CAD build for the part. Positions are in the model's coordinates, mm. A direction names the side the tool comes from. Round coordinates to 2 decimals unless told otherwise and drop trailing zeros. Write each loop counter-clockwise with the first axis right and the second up, starting at its lowest first coordinate (ties: lowest second). Pieces come first, ordered by that corner, then holes. Notation, with made-up numbers: (54.25, 57) - (62.25, 57) arc R30 ccw to (62.25, 94) - close; hole circle Ø5 at (-35, -18.5). An arc over 180 degrees is marked (long way). Answer in a Markdown table with one row per item.
```python
from build123d import *

# Parameters (mm, degrees)
F0_W     = 6.35
F0_H     = 38.1
F1_DEPTH = 25.4
F3_DEPTH = 12.5


with BuildPart() as f1:
    # F0 (on Top) → F1 (new body)
    with BuildSketch(Plane.XY):
        with Locations((-3.175, 0)):
            Rectangle(F0_W, F0_H)
    extrude(amount=F1_DEPTH)

    # F2 (on face) → F3 (join)
    with BuildSketch(Plane(origin=(-6.35, 0, 0), x_dir=(0, -1, 0), z_dir=(-1, 0, 0))):
        with BuildLine():
            Line((-19.05, 25.4), (-19.05, 19.05))
            ThreePointArc((-19.05, 19.05), (0, 0), (19.05, 19.05))
            Line((19.05, 19.05), (19.05, 25.4))
            Line((19.05, 25.4), (14, 25.4))
            Line((14, 25.4), (14, 19.05))
            ThreePointArc((14, 19.05), (0, 5.05), (-14, 19.05))
            Line((-14, 19.05), (-14, 25.4))
            Line((-14, 25.4), (-19.05, 25.4))
        make_face()
    extrude(amount=F3_DEPTH)


solid = f1.part
```
Q1. Saw through at C-C on z = 9.5. List the corners of the cut face in (x, y), then the cut area to 3 significant figures.
Computed:
| item | result |
|---|---|
| outline | (-18.85, -16.48) - (-6.35, -16.48) - (-6.35, -19.05) - (0, -19.05) - (0, 19.05) - (-6.35, 19.05) - (-6.35, 16.48) - (-18.85, 16.48) - (-18.85, 10.24) - (-6.35, 10.24) - (-6.35, -10.24) - (-18.85, -10.24) - close |
| area | 398 mm2 |
Q2. 3-axis set-ups, long thin cutter, end or side, ignore diameter. For faces 1 (the flat face through (-6.35, 14, 4)), 2 (the flat face through (-6.35, -15, 5)), 3 (the cylindrical face through (-13, 0, 0)), 4 (the cylindrical face through (-12.512, -0.308, 5.053)): which of +Z, -Z, +X, -X, +Y, -Y reach the whole face in a straight line?
Computed:
| item | result |
|---|---|
| face 1 | -Z, -X, +Y |
| face 2 | -Z, -X, -Y |
| face 3 | -Z, -X |
| face 4 | +Z, -X |
Q3. Saw through at D-D on z = 17.5. List the corners of the cut face in (x, y).
Computed:
| item | result |
|---|---|
| outline | (-18.85, -18.99) - (-6.35, -18.99) - (-6.35, -19.05) - (0, -19.05) - (0, 19.05) - (-6.35, 19.05) - (-6.35, 18.99) - (-18.85, 18.99) - (-18.85, 13.91) - (-6.35, 13.91) - (-6.35, -13.91) - (-18.85, -13.91) - close |
Q4. Saw through at B-B on x = -7.75. List the corners of the cut face in (y, z).
Computed:
| item | result |
|---|---|
| outline | (-19.05, 19.05) arc R19.05 ccw to (19.05, 19.05) - (19.05, 25.4) - (14, 25.4) - (14, 19.05) arc R14 cw to (-14, 19.05) - (-14, 25.4) - (-19.05, 25.4) - close |
Q5. Drill centre lines: line 1 (Y direction, x = -13, z = 20.5); line 2 (X direction, y = 7, z = 16); line 3 (Y direction, x = -10, z = 16). Where is each one in solid material? Low to high.
Computed:
| item | result |
|---|---|
| line 1 | y = -19.05 to -14, 14 to 19.05 |
| line 2 | x = -6.35 to 0 |
| line 3 | y = -18.8 to -13.66, 13.66 to 18.8 |
Q6. Saw through at A-A on y = -10. List the corners of the cut face in (x, z).
Computed:
| item | result |
|---|---|
| outline | (-18.85, 2.84) - (-6.35, 2.84) - (-6.35, 0) - (0, 0) - (0, 25.4) - (-6.35, 25.4) - (-6.35, 9.25) - (-18.85, 9.25) - close |
Q7. Flat gauge pins, fed straight in: pin 1 (5.5 mm diameter, centred on y = -6, z = 11, fed in from -X); pin 2 (12 mm diameter, centred on y = 4.5, z = 14.5, fed in from +X); pin 3 (3 mm diameter, centred on x = -15, y = 3, fed in from -Z); pin 4 (6 mm diameter, centred on x = -11.5, y = -3.5, fed in from +Z). Where does each tip first touch, or does it go through?
Computed:
| item | result |
|---|---|
| pin 1 | stops at x = -6.35 |
| pin 2 | stops at x = 0 |
| pin 3 | stops at z = 0.06 |
| pin 4 | stops at z = 6.65 |
